Geometry check sheet. Reference: the model listing, model coordinates, mm. A direction names the side the tool comes from. Give positions to 0.01 mm unless a question says otherwise; leave off trailing zeros. Write each loop counter-clockwise with the first axis right and the second up, starting at its lowest first coordinate (ties: lowest second). Pieces come first, ordered by that corner, then holes. Notation, with made-up numbers: (-23, 25) -> (25, 25) arc R23 cw to (25, 55) -> close; hole circle Ø4 at (50, 68.25). An arc over 180 degrees is marked (long way). Write item = value, one per line. Start each with the question number.
1. Mould release check, pull along X, two halves, no side actions. Record for faces 1 (the flat face through (35.933, 9.392, -85.592)), 2 (the flat face through (-36.653, 16.536, 57.394)), 3 (the flat face through (35.56, 12, 67)): pulls with the +X half, pulls with the -X half, needs draft (parallel to the pull), parting line crosses it, or undercut.
2. Set-up check for faces 4 (the flat face through (-17.336, 15.831, 74.948)), 5 (the flat face through (36.8, 15.8, -41.2)), 6 (the flat face through (29.34, 11.51, 63.59)): record each of +Z, -Z, +X, -X, +Y, -Y from which the full face is reachable in a straight line by a thin tool's end or side.
3. Cross-section at B-B, the plane z = 43. Record the cut outline in (x, y).
4. Cross-section at C-C, the plane z = 69.85. State how many separate pieces and enclosed holes the cut face has, plus the area to 3 significant figures.
5. Depth check by flat-ended pin: P1, Ø3.5, axis at y = 12.7, z = 69.85, coming from the -X side; P2, Ø3, axis at x = -32.5, y = 18, coming from the -Z side; P3, Ø12, axis at x = 3, z = -27.5, coming from the +Y side; P4, Ø10, axis at x = -5, y = 14.5, coming from the -Z side. Enter the tip coordinate at first touch or a pass-through.
6. Thickness scan on line 1 along X through (y, z) = (1.5, -3); line 2 along X through (y, z) = (6.5, -7); line 3 along X through (y, z) = (11, 61.5). Record the ranges inside material, lowest first.
7. Cross-section at A-A, the plane x = -5.5. Record the cut outline in (y, z).
```python
from build123d import *

# Parameters (mm, degrees)
BOSS_EXTRUDE1_DEPTH = 12.7
CUT_EXTRUDE3_DEPTH  = 77.2
SKETCH8_W           = 71.12
SKETCH8_H           = 101.6
BOSS_EXTRUDE3_DEPTH = 2.54
SKETCH9_W           = 14.4145
SKETCH9_H           = 99.06
SKETCH9_W_2         = 21.5265
SKETCH9_H_2         = 49.53
SKETCH9_W_3         = 16.637
SKETCH9_H_3         = 46.99
CUT_EXTRUDE4_DEPTH  = 2.54
BOSS_EXTRUDE4_DEPTH = 12.7
SKETCH19_W          = 2.54
SKETCH19_H          = 2.54
BOSS_EXTRUDE6_DEPTH = 25.4
BOSS_EXTRUDE7_DEPTH = 6.35
BOSS_EXTRUDE8_DEPTH = 6.35
CUT_EXTRUDE9_DEPTH  = 77.2
CUT_EXTRUDE10_DEPTH = 2.54
SKETCH28_W          = 12.7
SKETCH28_H          = 7.62
CUT_EXTRUDE11_DEPTH = 2.54
CUT_EXTRUDE12_DEPTH = 12.7
CUT_EXTRUDE13_DEPTH = 12.7
SKETCH32_R          = 2.032
CUT_EXTRUDE15_DEPTH = 77.2
SKETCH33_W          = 2.54
SKETCH33_H          = 2.54
BOSS_EXTRUDE9_DEPTH = 15.24
CUT_EXTRUDE17_DEPTH = 2.54


with BuildPart() as part:
    # Sketch1 → Boss-Extrude1 (new body)
    with BuildSketch(Plane(origin=(0, 0, 0), x_dir=(1, 0, 0), z_dir=(0, 1, 0))):
        Polygon((38.1, -76.2), (38.1, 76.2), (35.56, 76.2), (35.56, -57.367897552), (19.267897552, -73.66), (-19.267897552, -73.66), (-35.56, -57.367897552), (-35.56, 76.2), (-38.1, 76.2), (-38.1, -76.2), align=None)
        Polygon((-35.56, -73.66), (-22.86, -73.66), (-35.56, -60.96), align=None, mode=Mode.SUBTRACT)
        Polygon((22.86, -73.66), (35.56, -60.96), (35.56, -73.66), align=None, mode=Mode.SUBTRACT)
    extrude(amount=BOSS_EXTRUDE1_DEPTH)

    # Sketch7 → Cut-Extrude3 (cut, through all)
    with BuildSketch(Plane(origin=(38.1, 0, 0), x_dir=(0, 0, -1), z_dir=(1, 0, 0))):
        Polygon((-57.15, 10.16), (-10.795093656, 10.16), (-10.795093656, 5.095127003), align=None)
        Polygon((-57.15, 7.60488323), (-57.15, 2.54), (-10.795, 2.54), align=None)
        Polygon((-8.255093656, 10.16), (38.1, 10.16), (-8.255093656, 5.095106537), align=None)
        Polygon((-8.255, 2.54), (38.1, 2.54), (38.1, 7.60488323), align=None)
    extrude(amount=-CUT_EXTRUDE3_DEPTH, mode=Mode.SUBTRACT)

    # Sketch8 → Boss-Extrude3 (add)
    with BuildSketch(Plane.XZ):
        with Locations((0, -19.05)):
            Rectangle(SKETCH8_W, SKETCH8_H)
    extrude(amount=-BOSS_EXTRUDE3_DEPTH)

    # Sketch9 → Cut-Extrude4 (cut)
    with BuildSketch(Plane(origin=(0, 2.54, 0), x_dir=(1, 0, 0), z_dir=(0, 1, 0))):
        with Locations((-28.35275, 20.32)):
            Rectangle(SKETCH9_W, SKETCH9_H)
        with BuildLine():
            Line((-14.4145, 64.008), (-14.4145, -24.892))
            ThreePointArc((-14.4145, -24.892), (-16.51, -26.9875), (-18.6055, -24.892))
            Line((-18.6055, -24.892), (-18.6055, 64.008))
            ThreePointArc((-18.6055, 64.008), (-16.51, 66.1035), (-14.4145, 64.008))
        make_face()
        with Locations((24.79675, 45.085)):
            Rectangle(SKETCH9_W_2, SKETCH9_H_2)
        with Locations((-3.556, 43.815)):
            Rectangle(SKETCH9_W_3, SKETCH9_H_3)
        with BuildLine():
            Line((7.3025, 64.008), (7.3025, -24.892))
            ThreePointArc((7.3025, -24.892), (9.398, -26.9875), (11.4935, -24.892))
            Line((11.4935, -24.892), (11.4935, 64.008))
            ThreePointArc((11.4935, 64.008), (9.398, 66.1035), (7.3025, 64.008))
        make_face()
        with Locations((-3.556, -5.715)):
            Rectangle(SKETCH9_W_3, SKETCH9_H_3)
        with Locations((24.79675, -5.715)):
            Rectangle(SKETCH9_W_2, SKETCH9_H_3)
    extrude(amount=-CUT_EXTRUDE4_DEPTH, mode=Mode.SUBTRACT)

    # Sketch16 → Boss-Extrude4 (add)
    with BuildSketch(Plane.XZ):
        Polygon((-35.56, -76.2), (-31.75, -92.71), (31.75, -92.71), (35.56, -76.2), (38.1, -76.2), (33.703846154, -95.25), (-33.703846154, -95.25), (-38.1, -76.2), align=None)
    extrude(amount=-BOSS_EXTRUDE4_DEPTH)

    # Sketch19 → Boss-Extrude6 (add)
    with BuildSketch(Plane(origin=(0, 0, -69.85), x_dir=(-1, 0, 0), z_dir=(0, 0, -1))):
        with Locations((19.8755, 1.27)):
            Rectangle(SKETCH19_W, SKETCH19_H)
        with Locations((-12.7635, 1.27)):
            Rectangle(SKETCH19_W, SKETCH19_H)
    extrude(amount=BOSS_EXTRUDE6_DEPTH)

    # Sketch21 → Boss-Extrude7 (add)
    with BuildSketch(Plane(origin=(0, 12.7, 0), x_dir=(1, 0, 0), z_dir=(0, 1, 0))):
        Polygon((38.1, 38.1), (38.1, 76.2), (33.703846154, 95.25), (31.75, 92.71), (35.56, 76.2), (35.56, 38.1), align=None)
        Polygon((-35.56, 38.1), (-38.1, 38.1), (-38.1, 76.2), (-33.703846154, 95.25), (-31.75, 92.71), (-35.56, 76.2), align=None)
    extrude(amount=BOSS_EXTRUDE7_DEPTH)

    # Sketch24 → Boss-Extrude8 (add)
    with BuildSketch(Plane(origin=(0, 12.7, 0), x_dir=(1, 0, 0), z_dir=(0, 1, 0))):
        Polygon((-38.1, -57.367897552), (-38.1, -76.2), (-19.267897552, -76.2), (-15.457897552, -76.2), (-15.457897552, -73.66), (-19.267897552, -73.66), (-35.56, -57.367897552), (-35.56, -53.557897552), (-38.1, -53.557897552), align=None)
        Polygon((-22.86, -73.66), (-35.56, -60.96), (-35.56, -73.66), align=None, mode=Mode.SUBTRACT)
        Polygon((19.267897552, -76.2), (38.1, -76.2), (38.1, -57.367897552), (38.1, -53.557897552), (35.56, -53.557897552), (35.56, -57.367897552), (19.267897552, -73.66), (15.457897552, -73.66), (15.457897552, -76.2), align=None)
        Polygon((22.86, -73.66), (35.56, -60.96), (35.56, -73.66), align=None, mode=Mode.SUBTRACT)
    extrude(amount=BOSS_EXTRUDE8_DEPTH)

    # Sketch26 → Cut-Extrude9 (cut, through all)
    with BuildSketch(Plane(origin=(38.1, 0, 0), x_dir=(0, 0, -1), z_dir=(1, 0, 0))):
        Polygon((-53.557897552, 12.7), (-59.907897552, 19.05), (-53.557897552, 19.05), align=None)
        Polygon((-59.907897552, 0), (-66.257897552, 6.35), (-76.2, 6.35), (-76.2, 0), align=None)
    extrude(amount=-CUT_EXTRUDE9_DEPTH, mode=Mode.SUBTRACT)

    # Sketch27 → Cut-Extrude10 (cut)
    with BuildSketch(Plane.XY.offset(76.2)):
        Polygon((-15.457897552, 12.7), (-19.267897552, 19.05), (-15.457897552, 19.05), align=None)
        Polygon((15.457897552, 12.7), (15.457897552, 19.05), (19.267897552, 19.05), align=None)
        Polygon((-19.267897552, 6.35), (-15.457897552, 10.16), (15.457897552, 10.16), (19.267897552, 6.35), align=None)
    extrude(amount=-CUT_EXTRUDE10_DEPTH, mode=Mode.SUBTRACT)

    # Sketch28 → Cut-Extrude11 (cut)
    with BuildSketch(Plane.XY.offset(76.2)):
        with Locations((-29.21, 12.7)):
            Rectangle(SKETCH28_W, SKETCH28_H)
        with Locations((29.21, 12.7)):
            Rectangle(SKETCH28_W, SKETCH28_H)
    extrude(amount=-CUT_EXTRUDE11_DEPTH, mode=Mode.SUBTRACT)

    # Sketch29 → Cut-Extrude12 (cut)
    with BuildSketch(Plane(origin=(38.1, 0, 0), x_dir=(0, 0, -1), z_dir=(1, 0, 0))):
        Polygon((38.1, 12.7), (44.45, 19.05), (38.1, 19.05), align=None)
        Polygon((40.64, 0), (46.99, 6.35), (76.2, 6.35), (92.71, 0), align=None)
        Polygon((76.2, 19.05), (92.71, 12.7), (95.25, 12.7), (95.25, 19.05), align=None)
    extrude(amount=-CUT_EXTRUDE12_DEPTH, mode=Mode.SUBTRACT)

    # Sketch30 → Cut-Extrude13 (cut)
    with BuildSketch(Plane.ZY.offset(38.1)):
        Polygon((-38.1, 12.7), (-44.45, 19.05), (-38.1, 19.05), align=None)
        Polygon((-46.99, 6.35), (-40.64, 0), (-92.71, 0), (-76.2, 6.35), align=None)
        Polygon((-76.2, 19.05), (-92.71, 12.7), (-95.25, 12.7), (-95.25, 19.05), align=None)
    extrude(amount=-CUT_EXTRUDE13_DEPTH, mode=Mode.SUBTRACT)

    # Sketch32 → Cut-Extrude15 (cut, through all)
    with BuildSketch(Plane(origin=(38.1, 0, 0), x_dir=(0, 0, -1), z_dir=(1, 0, 0))):
        with Locations((45.72, 12.7)):
            Circle(SKETCH32_R)
        with Locations((53.34, 12.7)):
            Circle(SKETCH32_R)
        with Locations((60.96, 12.7)):
            Circle(SKETCH32_R)
        with Locations((68.58, 12.7)):
            Circle(SKETCH32_R)
        with Locations(Location((-69.85, 12.7, 0), (0, 0, 180))):  # turned: the seam where the file's is
            Circle(SKETCH32_R)
    extrude(amount=-CUT_EXTRUDE15_DEPTH, mode=Mode.SUBTRACT)

    # Sketch33 → Boss-Extrude9 (add)
    with BuildSketch(Plane.ZY.offset(21.1455)):
        with Locations((-19.05, 1.27)):
            Rectangle(SKETCH33_W, SKETCH33_H)
    extrude(amount=BOSS_EXTRUDE9_DEPTH)

    # Sketch35 → Cut-Extrude17 (cut)
    with BuildSketch(Plane.XY.offset(-92.71)):
        Polygon((-31.75, 12.7), (-21.59, 7.62), (21.59, 7.62), (31.75, 12.7), align=None)
    extrude(amount=-CUT_EXTRUDE17_DEPTH, mode=Mode.SUBTRACT)


solid = part.part
```
Answers:
q1.face_1 = pulls with the +X half
q1.face_2 = needs draft
q1.face_3 = undercut
q2.face_4 = +Z, -Z, +Y
q2.face_5 = +X, -X, +Y
q2.face_6 = +Y, -Y
q3.outline = (-38.1, 0) -> (-35.56, 0) -> (-35.56, 2.54) -> (-38.1, 2.54) -> close; (-38.1, 6.06) -> (-35.56, 6.06) -> (-35.56, 8.61) -> (-38.1, 8.61) -> close; (-38.1, 10.16) -> (-35.56, 10.16) -> (-35.56, 12.7) -> (-38.1, 12.7) -> close; (35.56, 0) -> (38.1, 0) -> (38.1, 2.54) -> (35.56, 2.54) -> close; (35.56, 6.06) -> (38.1, 6.06) -> (38.1, 8.61) -> (35.56, 8.61) -> close; (35.56, 10.16) -> (38.1, 10.16) -> (38.1, 12.7) -> (35.56, 12.7) -> close
q4.separate_pieces = 8
q4.enclosed_holes = 0
q4.area = 106 mm^2
q5.P1 = through
q5.P2 = 58.93
q5.P3 = 2.54
q5.P4 = 73.66
q6.line_1 = -38.1 to -35.56, -21.15 to -18.61, -14.41 to -11.87, 4.76 to 7.3, 11.49 to 14.03, 35.56 to 38.1
q6.line_2 = -38.1 to -35.56, 35.56 to 38.1
q6.line_3 = -38.1 to -35.56, -35.02 to -31.43, 31.43 to 35.02, 35.56 to 38.1
q7.outline = (0, -95.25) -> (7.62, -95.25) -> (7.62, -92.71) -> (0, -92.71) -> close; (0, -69.85) -> (2.54, -69.85) -> (2.54, -67.31) -> (0, -67.31) -> close; (0, -20.32) -> (2.54, -20.32) -> (2.54, -17.78) -> (0, -17.78) -> close; (0, 29.21) -> (2.54, 29.21) -> (2.54, 31.75) -> (0, 31.75) -> close; (10.16, 73.66) -> (12.7, 73.66) -> (12.7, 76.2) -> (10.16, 76.2) -> close
